```python
from build123d import *

# Parameters (mm, degrees)
FILLET_1_R          = 2
FILLET_2_R          = 70
SKETCH_2_R          = 11
CUT_EXTRUDE_1_DEPTH = 130.302519771


with BuildPart() as part:
    # Эскиз1 → Повернуть1 (revolve)
    with BuildSketch(Plane.XY, mode=Mode.PRIVATE) as revolve_1_sk:
        Polygon((0, 0), (17.5, 0), (14.5, -20), (16.5, -63.5), (14.5, -107), (17.5, -127), (0, -127), align=None)
    revolve(revolve_1_sk.sketch.rotate(Axis((0, 24.4253472, 0), (0, -1, 0)), 90), axis=Axis((0, 24.4253472, 0), (0, -1, 0)))

    # Скругление1
    fillet_1_edges = [part.edges().sort_by_distance(p)[0] for p in [
        (0, 0, -17.5),
        (0, -127, -17.5),
    ]]
    fillet(fillet_1_edges, radius=FILLET_1_R)

    # Скругление2
    # the kernel refuses this fillet: 70 mm, written as the material it adds along each edge
    with BuildSketch(Plane(origin=(0, -20, 0), x_dir=(0, 0, 1), z_dir=(1, 0, 0))) as fillet_2_piece_1:
        with BuildLine():
            CenterArc((14.5 + FILLET_2_R * 1.00343316746, FILLET_2_R * 0.0516950223501), FILLET_2_R, 177.367565131, 11.163200479)
            Line((14.5 + FILLET_2_R * 0.00448843750259, FILLET_2_R * 0.0976235156813), (14.5 - FILLET_2_R * 0.0154904570965, FILLET_2_R * 0.0985420855479))
            Line((14.5 - FILLET_2_R * 0.0154904570965, FILLET_2_R * 0.0985420855479), (14.5 - FILLET_2_R * 0.0200686633491, -FILLET_2_R * 0.001033900447))
            Line((14.5 - FILLET_2_R * 0.0200686633491, -FILLET_2_R * 0.001033900447), (14.5 - FILLET_2_R * 0.00528191247035, -FILLET_2_R * 0.0996122396387))
            Line((14.5 - FILLET_2_R * 0.00528191247035, -FILLET_2_R * 0.0996122396387), (14.5 + FILLET_2_R * 0.014496814587, -FILLET_2_R * 0.0966454305801))
        make_face()
    revolve(axis=Axis((0, -20, 0), (0, -1, 0)))
    with BuildSketch(Plane(origin=(0, -107, 0), x_dir=(0, 0, 1), z_dir=(1, 0, 0))) as fillet_2_piece_2:
        with BuildLine():
            CenterArc((14.5 + FILLET_2_R * 1.00343316746, -FILLET_2_R * 0.0516950223501), FILLET_2_R, 171.46923439, 11.163200479)
            Line((14.5 + FILLET_2_R * 0.014496814587, FILLET_2_R * 0.0966454305801), (14.5 - FILLET_2_R * 0.00528191247035, FILLET_2_R * 0.0996122396387))
            Line((14.5 - FILLET_2_R * 0.00528191247035, FILLET_2_R * 0.0996122396387), (14.5 - FILLET_2_R * 0.0200686633491, FILLET_2_R * 0.001033900447))
            Line((14.5 - FILLET_2_R * 0.0200686633491, FILLET_2_R * 0.001033900447), (14.5 - FILLET_2_R * 0.0154904570965, -FILLET_2_R * 0.0985420855479))
            Line((14.5 - FILLET_2_R * 0.0154904570965, -FILLET_2_R * 0.0985420855479), (14.5 + FILLET_2_R * 0.00448843750259, -FILLET_2_R * 0.0976235156813))
        make_face()
    revolve(axis=Axis((0, -107, 0), (0, -1, 0)))
    # the kernel refuses this fillet: 70 mm, written as the material it takes off along each edge
    with BuildSketch(Plane(origin=(0, -63.5, 0), x_dir=(0, 0, 1), z_dir=(1, 0, 0))) as fillet_2_2_piece_1:
        with BuildLine():
            CenterArc((16.5 - FILLET_2_R * 1.00105638482, 0), FILLET_2_R, 357.367565131, 5.264869738)
            Line((16.5 - FILLET_2_R * 0.0021116548658, FILLET_2_R * 0.0459284933312), (16.5 + FILLET_2_R * 0.0178672397333, FILLET_2_R * 0.0468470631978))
            Line((16.5 + FILLET_2_R * 0.0178672397333, FILLET_2_R * 0.0468470631978), (16.5 + FILLET_2_R * 0.0200211276964, 0))
            Line((16.5 + FILLET_2_R * 0.0200211276964, 0), (16.5 + FILLET_2_R * 0.0178672397333, -FILLET_2_R * 0.0468470631978))
            Line((16.5 + FILLET_2_R * 0.0178672397333, -FILLET_2_R * 0.0468470631978), (16.5 - FILLET_2_R * 0.0021116548658, -FILLET_2_R * 0.0459284933312))
        make_face()
    revolve(axis=Axis((0, -63.5, 0), (0, -1, 0)), mode=Mode.SUBTRACT)

    # Эскиз2 → Вырез-Вытянуть1 (cut, through all)
    with BuildSketch(Plane(origin=(0, 0, 0), x_dir=(1, 0, 0), z_dir=(0, 1, 0))):
        with Locations(Location((0, 0, 0), (0, 0, 270))):
            Circle(SKETCH_2_R)
    extrude(amount=-CUT_EXTRUDE_1_DEPTH, mode=Mode.SUBTRACT)


solid = part.part
```
The model under review builds one solid part; all positions refer to its coordinate system, in mm. A direction names the side the tool comes from. Round coordinates to 2 decimals unless told otherwise and drop trailing zeros. Loops run counter-clockwise (first coordinate to the right, second up) from the corner with the lowest first, then second, coordinate; pieces in that order, holes last.
Item 1: For faces 1 (the face through (13.815, -83.675, 7.186)), 2 (the face through (-5, -127, 10)), list the 3-axis set-ups (+Z, -Z, +X, -X, +Y, -Y) from which the entire face can be reached by the end or side of a thin tool; tool diameter is ignored.
Determined:
face 1: none
face 2: +Z, -Z, +X, -X, -Y
Item 2: Clearance check with flat-ended pins moving along their axes: pin 1 Ø1.5 at (y, z) = (-12.5, 3.5) entering from -X; pin 2 Ø5 at (y, z) = (-66, 0) entering from -X; pin 3 Ø1.5 at (y, z) = (-70, 5) entering from +X; pin 4 Ø1.5 at (x, z) = (-6.5, -8) entering from +Y. State where each tip first meets the part, or that it passes through.
Determined:
pin 1: stops at x = -15.42
pin 2: stops at x = -16.43
pin 3: stops at x = 15.64
pin 4: stops at y = 0
Item 3: Take a section at A-A (y = -56). Write out the cut boundary in (x, z).
Determined:
outline: circle Ø32.31 at (0, 0); hole circle Ø22 at (0, 0)
Item 4: Take a section at B-B (y = -16.5). Write out the cut boundary in (x, z).
Determined:
outline: circle Ø30.21 at (0, 0); hole circle Ø22 at (0, 0)
Item 5: Mouldability with a two-part tool opening along Z and no side actions: class faces 3 (the face through (15.58, -10.27, -3.46)), 4 (the face through (-5, 0, -10)), 5 (the face through (-10.74, -62.61, -2.38)) as released by +Z, released by -Z, zero draft, split by the parting line, or undercut.
Determined:
face 3: split by the parting line
face 4: zero draft
face 5: undercut
Item 6: For line 1 (X direction, y = -120, z = 8); line 2 (Z direction, x = 7.5, y = -31); line 3 (X direction, y = -38, z = 0), list the stretches that pass through material, from the lowest coordinate up.
Determined:
line 1: x = -14.37 to -7.55, 7.55 to 14.37
line 2: z = -13 to -8.05, 8.05 to 13
line 3: x = -15.33 to -11, 11 to 15.33
